Job drawing, mm, ordinate dimensions from the low corner. One solid piece. A direction names the side the tool comes from. Coordinates: 2 decimals unless noted, no trailing zeros. Order: outer loops, then holes, each group sorted by start corner. A loop starts at its lowest first (then second) coordinate and runs counter-clockwise, first axis right, second up. Notation, with made-up numbers: (17, -24.75) - (26, -24.75) arc R16 cw to (26, 4.25) - close; hole circle Ø9 at (-37, -36). An arc over 180 degrees is marked (long way). Return JSON: item names as keys, results as strings.
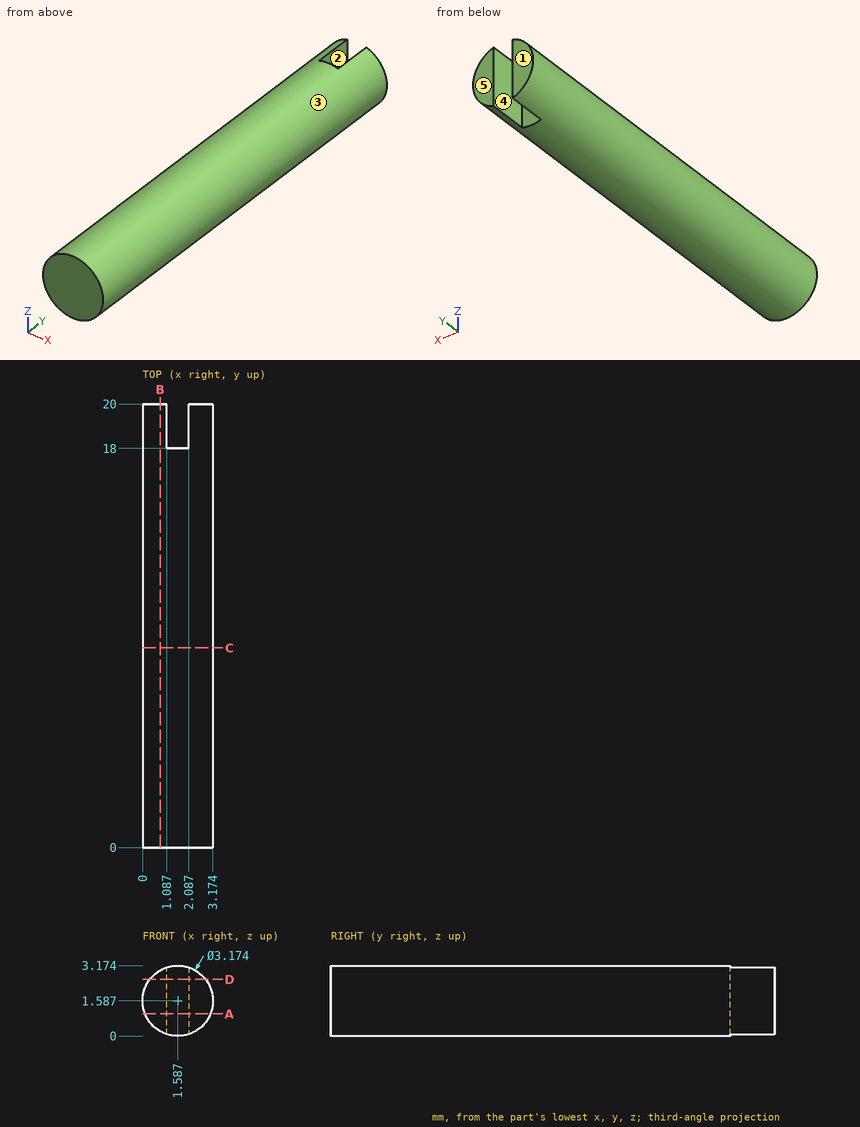
1. Mould opens along X. For the marked faces 3, 4 and 5 say: pulls with the +X half, pulls with the -X half, needs draft (parallel to the pull), parting line crosses it, or undercut.
Check values:
{"face 3": "parting line crosses it", "face 4": "undercut", "face 5": "needs draft"}
2. Cut at A-A on z = 1. Give the cut face in (x, y), plus the area to 3 significant figures.
Check values:
{"outline": "(0.11, 0) - (3.06, 0) - (3.06, 20) - (2.09, 20) - (2.09, 18) - (1.09, 18) - (1.09, 20) - (0.11, 20) - close", "area": "57.0 mm²"}
3. Cut at D-D on z = 2.55. Give the cut face in (x, y), plus the area to 3 significant figures.
Check values:
{"outline": "(0.33, 0) - (2.85, 0) - (2.85, 20) - (2.09, 20) - (2.09, 18) - (1.09, 18) - (1.09, 20) - (0.33, 20) - close", "area": "48.5 mm²"}
4. Tool access for the marked faces 1 and 2: list every direction of +Z, -Z, +X, -X, +Y, -Y with a clear straight run to the whole face (end or side of a thin tool).
Check values:
{"face 1": "+Z, -Z, +X, -X, +Y", "face 2": "+Z, -Z, +Y"}
5. Cut at C-C on y = 9. Give the cut face in (x, z).
Check values:
{"outline": "circle Ø3.17 at (1.59, 1.59)"}
6. Probe L1, parallel to X at y = 18.25, z = 1.6; L2, parallel to Y at x = 1.4, z = 2.95; L3, parallel to X at y = 2.75, z = 1.5. List the from-to ranges inside material, lowest first.
Check values:
{"L1": "0 to 1.09, 2.09 to 3.17", "L2": "0 to 18", "L3": "0 to 3.17"}
7. Cut at B-B on x = 0.8. Give the cut face in (y, z), plus the area to 3 significant figures.
Check values:
{"outline": "(0, 0.21) - (20, 0.21) - (20, 2.97) - (0, 2.97) - close", "area": "55.1 mm²"}
